Can you work these out from the model? Positions are in its coordinate system, mm. Face numbers are marked on the shaded views. A direction names the side the tool comes from. Coordinates: 2 decimals unless noted, no trailing zeros. Order: outer loops, then holes, each group sorted by start corner. A loop starts at its lowest first (then second) coordinate and runs counter-clockwise, first axis right, second up. Notation, with made-up numbers: (-36.5, 36) -> (13.5, 36) arc R20 cw to (13.5, 64) -> close; hole circle Ø3 at (-37.5, 21). An arc over 180 degrees is marked (long way). Use a Markdown table: item, result. Add a question column.
1. Suppose I cut it at C-C, the plane y = 26. List the corners of the cut face in (x, z) for me, then the cut area to 3 significant figures.
2. For pin 1 Ø12 at (x, z) = (-5.5, -3.5) entering from -Y; pin 2 Ø12 at (x, y) = (5.5, 10) entering from -Z; pin 3 Ø5 at (x, y) = (0.5, 11.5) entering from -Z; pin 4 Ø1.6 at (x, z) = (0, -5.5) entering from +Y, each with a flat end and sliding along its axis, tell me the tip position at first contact or that it passes through.
3. Suppose I cut it at B-B, the plane z = 0. List the corners of the cut face in (x, y) for me.
4. Suppose I cut it at A-A, the plane y = 35.5. List the corners of the cut face in (x, z) for me, then the cut area to 3 significant figures.
5. For the marked faces 1, 2, 3, 4 and 5, which set-ups out of +Z, -Z, +X, -X, +Y, -Y let a thin tool reach every point of the face, with its end or its side?
6. If I drill on line 1 along X through (y, z) = (7, 3); line 2 along X through (y, z) = (6, 4.5); line 3 along Y through (x, z) = (-4, -1.5), over which ranges is the centre line in solid material (lowest first)? Write a range as from..to.
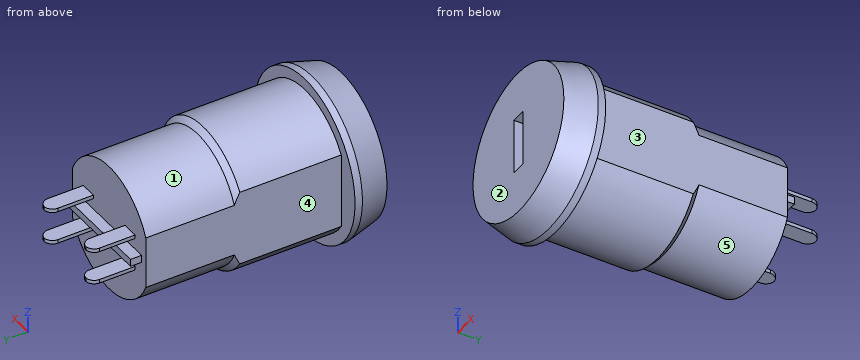
```python
from build123d import *

# Parameters (mm, degrees)
SKETCH_1_R          = 11
EXTRUDE_1_DEPTH     = 5
CHAMFER_1_SIZE      = 4
CHAMFER_1_SIZE2     = 1.07179677
EXTRUDE_3_DEPTH     = 26.5
SKETCH_4_W          = 2
SKETCH_4_H          = 7.5
CUT_EXTRUDE_1_DEPTH = 10
SKETCH_6_W          = 2.2
SKETCH_6_H          = 0.5
EXTRUDE_1_2_DEPTH   = 6
SKETCH_7_W          = 14.2
SKETCH_7_H          = 1
EXTRUDE_2_DEPTH     = 1.5
CUT_EXTRUDE_START   = -12
SKETCH_9_R          = 9.5
SKETCH_9_R_2        = 8.75
CUT_EXTRUDE_2_DEPTH = 12
CHAMFER_2_SIZE      = 0.75
FILLET_1_R          = 1.2


# Some blends are built 0.0001 mm under size
with BuildPart() as part:
    # 草图1 → Extrude 1 (new body)
    with BuildSketch(Plane(origin=(0, 0, 0), x_dir=(1, 0, 0), z_dir=(0, 1, 0))):
        with Locations(Location((0, 0, 0), (0, 0, 270))):
            Circle(SKETCH_1_R)
    extrude(amount=EXTRUDE_1_DEPTH)

    # 倒角1
    chamfer_1_edges = [part.edges().sort_by_distance(p)[0] for p in [
        (0, 0, -11),
    ]]
    chamfer_1_side = [part.faces().sort_by_distance(p)[0] for p in [
        (0, 2.5, -11),
    ]]
    chamfer(chamfer_1_edges, length=CHAMFER_1_SIZE, length2=CHAMFER_1_SIZE2, reference=chamfer_1_side[0])

    # 草图3 → 拉伸3 (add)
    with BuildSketch(Plane(origin=(0, 5, 0), x_dir=(-1, 0, 0), z_dir=(0, 1, 0))):
        with BuildLine():
            Line((-8, 5.123475383), (-8, -5.123475383))
            ThreePointArc((-8, -5.123475383), (0, -9.5), (8, -5.123475383))
            Line((8, -5.123475383), (8, 5.123475383))
            ThreePointArc((8, 5.123475383), (0, 9.5), (-8, 5.123475383))
        make_face()
    extrude(amount=EXTRUDE_3_DEPTH)

    # 草图4 → 切除-拉伸1 (cut)
    with BuildSketch(Plane(origin=(0, 0, 0), x_dir=(-1, 0, 0), z_dir=(0, 1, 0))):
        Rectangle(SKETCH_4_W, SKETCH_4_H)
    extrude(amount=CUT_EXTRUDE_1_DEPTH, mode=Mode.SUBTRACT)

    # 草图6 → Extrude 1 2 (add)
    with BuildSketch(Plane(origin=(0, 31.5, 0), x_dir=(1, 0, 0), z_dir=(0, 1, 0))):
        with Locations((4.55, 2.25)):
            Rectangle(SKETCH_6_W, SKETCH_6_H)
        with Locations((-4.55, 2.25)):
            Rectangle(SKETCH_6_W, SKETCH_6_H)
        with Locations((4.55, -2.25)):
            Rectangle(SKETCH_6_W, SKETCH_6_H)
        with Locations((-4.55, -2.25)):
            Rectangle(SKETCH_6_W, SKETCH_6_H)
    extrude(amount=EXTRUDE_1_2_DEPTH)

    # 草图7 → 凸台-拉伸2 (add)
    with BuildSketch(Plane(origin=(0, 31.5, 0), x_dir=(1, 0, 0), z_dir=(0, 1, 0))):
        Rectangle(SKETCH_7_W, SKETCH_7_H)
    extrude(amount=EXTRUDE_2_DEPTH)

    # 草图9 → 切除-拉伸2 (cut)
    with BuildSketch(Plane(origin=(0, 31.5, 0), x_dir=(1, 0, 0), z_dir=(0, 1, 0)).offset(CUT_EXTRUDE_START)):
        Circle(SKETCH_9_R)
        Circle(SKETCH_9_R_2, mode=Mode.SUBTRACT)
    extrude(amount=CUT_EXTRUDE_2_DEPTH, mode=Mode.SUBTRACT)

    # 倒角2
    chamfer_2_edges = [part.edges().sort_by_distance(p)[0] for p in [
        (0, 19.5, 9.5),
        (0, 19.5, -9.5),
    ]]
    chamfer(chamfer_2_edges, length=CHAMFER_2_SIZE - 0.0001)  # a hair under: the kernel refuses the full size

    # 圆角1
    # the kernel refuses this fillet: 1.2 mm, written as the material it takes off along each edge
    with BuildSketch(Plane(origin=(-3.45, 37.5, -5.5), x_dir=(0, -1, 0), z_dir=(0, 0, 1)), Plane(origin=(-5.65, 37.5, 1), x_dir=(0, -1, 0), z_dir=(0, 0, -1)), Plane(origin=(5.65, 37.5, -1), x_dir=(0, -1, 0), z_dir=(0, 0, 1)), Plane(origin=(3.45, 37.5, 5.5), x_dir=(0, -1, 0), z_dir=(0, 0, -1))) as fillet_1_piece_1:
        with BuildLine():
            CenterArc((FILLET_1_R, -FILLET_1_R), FILLET_1_R, 90, 90)
            Line((0, -FILLET_1_R), (0, 0))
            Line((0, 0), (FILLET_1_R, 0))
        make_face()
    extrude(amount=6.5, mode=Mode.SUBTRACT)
    with BuildSketch(Plane(origin=(3.45, 37.5, -5.5), x_dir=(0, -1, 0), z_dir=(0, 0, 1)), Plane(origin=(5.65, 37.5, 1), x_dir=(0, -1, 0), z_dir=(0, 0, -1)), Plane(origin=(-5.65, 37.5, -1), x_dir=(0, -1, 0), z_dir=(0, 0, 1)), Plane(origin=(-3.45, 37.5, 5.5), x_dir=(0, -1, 0), z_dir=(0, 0, -1))) as fillet_1_piece_2:
        with BuildLine():
            CenterArc((FILLET_1_R, FILLET_1_R), FILLET_1_R, 180, 90)
            Line((0, FILLET_1_R), (0, 0))
            Line((0, 0), (FILLET_1_R, 0))
        make_face()
    extrude(amount=6.5, mode=Mode.SUBTRACT)


solid = part.part
```
Worked out:
| question | item | result |
|---|---|---|
| 1 | outline | (-8, -3.54) arc R8.75 ccw to (8, -3.54) -> (8, 3.54) arc R8.75 ccw to (-8, 3.54) -> close |
| 1 | area | 233 mm² |
| 2 | pin 1 | stops at y = 0 |
| 2 | pin 2 | stops at z = -10.78 |
| 2 | pin 3 | stops at z = -9.5 |
| 2 | pin 4 | stops at y = 31.5 |
| 3 | outline | (-11, 4) -> (-9.93, 0) -> (-1, 0) -> (-1, 10) -> (1, 10) -> (1, 0) -> (9.93, 0) -> (11, 4) -> (11, 5) -> (8, 5) -> (8, 31.5) -> (7.1, 31.5) -> (7.1, 33) -> (-7.1, 33) -> (-7.1, 31.5) -> (-8, 31.5) -> (-8, 5) -> (-11, 5) -> close |
| 4 | outline | (-5.65, -2.5) -> (-3.45, -2.5) -> (-3.45, -2) -> (-5.65, -2) -> close; (-5.65, 2) -> (-3.45, 2) -> (-3.45, 2.5) -> (-5.65, 2.5) -> close; (3.45, -2.5) -> (5.65, -2.5) -> (5.65, -2) -> (3.45, -2) -> close; (3.45, 2) -> (5.65, 2) -> (5.65, 2.5) -> (3.45, 2.5) -> close |
| 4 | area | 4.40 mm² |
| 5 | face 1 | +Z, +Y |
| 5 | face 2 | +Z, -Z, +X, -X, -Y |
| 5 | face 3 | +Z, -Z, +X, +Y |
| 5 | face 4 | +Z, -Z, -X, +Y |
| 5 | face 5 | -Z, +Y |
| 6 | line 1 | x = -8..-1, 1..8 |
| 6 | line 2 | x = -8..8 |
| 6 | line 3 | y = 0..31.5 |
